Read the model definition and answer for the solid it produces. Units are mm, in the model's axes. Face numbers are marked on the shaded views. A direction names the side the tool comes from. Give positions to 0.01 mm unless a question says otherwise; leave off trailing zeros. Loops run counter-clockwise (first coordinate to the right, second up) from the corner with the lowest first, then second, coordinate; pieces in that order, holes last. Notation, with made-up numbers: (82.5, 14) -> (114.5, 14) arc R23 cw to (114.5, 30) -> close; hole circle Ø4 at (-5, 36). An arc over 180 degrees is marked (long way). Return JSON: item names as keys, results as strings. Group by question number.
from build123d import *

# Parameters (mm, degrees)
F0_W     = 60
F0_H     = 50
F1_DEPTH = 5
F2_W     = 37.5
F2_H     = 50
F3_DEPTH = 30
F4_R     = 6
F5_DEPTH = 37.5
F6_W     = 37.5
F6_H     = 50
F7_DEPTH = 12.5


with BuildPart() as f1:
    # F0 (on Top) → F1 (new body)
    with BuildSketch(Plane.XY):
        Rectangle(F0_W, F0_H)
        with BuildLine():
            Line((-22.5574357373, -19.3509999587), (-12.5574357373, -19.3509999587))
            ThreePointArc((-12.5574357373, -19.3509999587), (-10.85, -21), (-12.5574357373, -22.6490000413))
            Line((-12.5574357373, -22.6490000413), (-22.5574357373, -22.6490000413))
            Line((-22.5574357373, -22.6490000413), (-24.9425642627, -22.6490000413))
            ThreePointArc((-24.9425642627, -22.6490000413), (-26.6490000413, -21.0574357373), (-25.0574357373, -19.3509999587))
            ThreePointArc((-25.0574357373, -19.3509999587), (-25, -19.35), (-24.9425642627, -19.3509999587))
            Line((-24.9425642627, -19.3509999587), (-22.5574357373, -19.3509999587))
        make_face(mode=Mode.SUBTRACT)
        with BuildLine():
            ThreePointArc((-12.4425642627, -0.6490000413), (-12.5, -0.65), (-12.5574357373, -0.6490000413))
            Line((-12.5574357373, -0.6490000413), (-24.9425642627, -0.6490000413))
            ThreePointArc((-24.9425642627, -0.6490000413), (-25, -0.65), (-25.0574357373, -0.6490000413))
            ThreePointArc((-25.0574357373, -0.6490000413), (-26.6490000413, 1.0574357373), (-24.9425642627, 2.6490000413))
            Line((-24.9425642627, 2.6490000413), (-12.5574357373, 2.6490000413))
            ThreePointArc((-12.5574357373, 2.6490000413), (-12.5, 2.65), (-12.4425642627, 2.6490000413))
            ThreePointArc((-12.4425642627, 2.6490000413), (-10.85, 1), (-12.4425642627, -0.6490000413))
        make_face(mode=Mode.SUBTRACT)
    extrude(amount=F1_DEPTH)

    # F2 (on Top) → F3 (join)
    with BuildSketch(Plane.XY):
        with Locations((18.75, 0)):
            Rectangle(F2_W, F2_H)
    extrude(amount=F3_DEPTH)

    # F4 (on face) → F5 (cut, through all)
    with BuildSketch(Plane.YZ.offset(37.5)):
        with Locations((-10, 17.5)):
            Circle(F4_R)
    extrude(amount=-F5_DEPTH, mode=Mode.SUBTRACT)

    # F6 (on face) → F7 (cut)
    with BuildSketch(Plane.XY.offset(30)):
        with Locations((18.75, 0)):
            Rectangle(F6_W, F6_H)
    extrude(amount=-F7_DEPTH, mode=Mode.SUBTRACT)


solid = f1.part
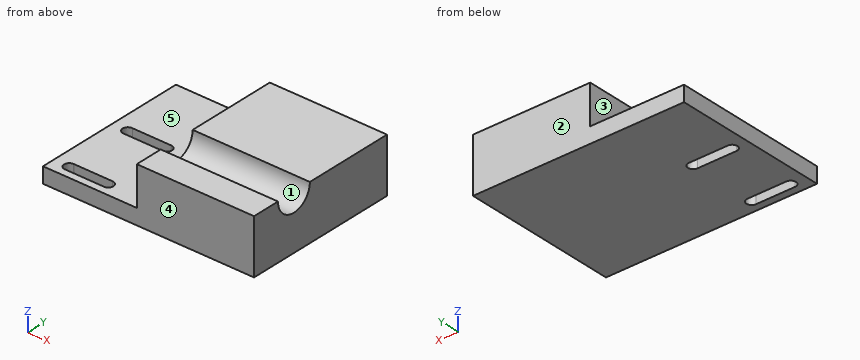
1. Flat-ended cylindrical pins translate along their axes: pin 1 Ø3 at (y, z) = (-17.5, 14.5) entering from -X; pin 2 Ø24 at (x, y) = (-18, 11) entering from +Z. Find the tip coordinate at first contact, or state that the pin passes through.
2. Straight lines are drawn through the part: line 1 (Y direction, x = -13, z = 3.5); line 2 (X direction, y = 1, z = 5.25); line 3 (Z direction, x = -16, y = -13.5). For each, find the intervals that lie inside material, in ascending order. Write a range as from..to.
3. Section B-B on y = -21 is taken. Determine the outline of the cut face in (x, z).
4. Determine the mould class of the marked faces 1, 2 and 3 for opening direction Y: pulls with the +Y half, pulls with the -Y half, needs draft (parallel to the pull), parting line crosses it, or undercut.
5. Section A-A on x = -20 is taken. Determine the outline of the cut face in (y, z), then the cut area to 3 significant figures.
6. Which of the six approach directions +Z, -Z, +X, -X, +Y, -Y give full straight-line access (tool end or side, diameter ignored) to the marked faces 4 and 5?
7. Section C-C on z = 3.5 is taken. Determine the outline of the cut face in (x, y), then the cut area to 3 significant figures.
8. Section D-D on y = -10 is taken. Determine the outline of the cut face in (x, z).
Completed:
{
 "1": {"pin 1": "stops at x = 0", "pin 2": "stops at z = 5"},
 "2": {"line 1": "y = -25..-22.65, -19.35..-0.65, 2.65..25", "line 2": "x = 0..37.5", "line 3": "z = 0..5"},
 "3": {"outline": "(-30, 0) -> (-26.65, 0) -> (-26.65, 5) -> (-30, 5) -> close; (-10.85, 0) -> (37.5, 0) -> (37.5, 17.5) -> (0, 17.5) -> (0, 5) -> (-10.85, 5) -> close"},
 "4": {"face 1": "undercut", "face 2": "pulls with the +Y half", "face 3": "needs draft"},
 "5": {"outline": "(-25, 0) -> (-22.65, 0) -> (-22.65, 5) -> (-25, 5) -> close; (-19.35, 0) -> (-0.65, 0) -> (-0.65, 5) -> (-19.35, 5) -> close; (2.65, 0) -> (25, 0) -> (25, 5) -> (2.65, 5) -> close", "area": "217 mm²"},
 "6": {"face 4": "+Z, -Z, +X, -X, -Y", "face 5": "+Z, -X, +Y, -Y"},
 "7": {"outline": "(-30, -25) -> (37.5, -25) -> (37.5, 25) -> (-30, 25) -> close; hole (-24.94, -22.65) -> (-12.56, -22.65) arc R1.65 ccw (long way) to (-12.56, -19.35) -> (-24.94, -19.35) arc R1.65 ccw (long way) to start; hole (-24.94, -0.65) -> (-12.56, -0.65) arc R1.65 ccw (long way) to (-12.56, 2.65) -> (-24.94, 2.65) arc R1.65 ccw (long way) to start", "area": "3,280 mm²"},
 "8": {"outline": "(-30, 0) -> (37.5, 0) -> (37.5, 11.5) -> (0, 11.5) -> (0, 5) -> (-30, 5) -> close"}
}
